Job drawing, mm, ordinate dimensions from the low corner. One solid piece. Give positions to 0.01 mm unless a question says otherwise; leave off trailing zeros. Order: outer loops, then holes, each group sorted by start corner. A loop starts at its lowest first (then second) coordinate and runs counter-clockwise, first axis right, second up. Notation, with made-up numbers: M 9,40.25 L 65,40.25 A12 ccw 65,45.25 Z; hole C -1.75,11.5 d1. An arc over 180 degrees is marked long. Put each result on its own line as item: value. Start each with the question number.
1) Drill centre lines: line 1 (Y direction, x = 46.5, z = 0.85); line 2 (X direction, y = 76, z = 0.4); line 3 (Y direction, x = 80, z = 0.75). Where is each one in solid material? Low to high. Write a range as [from, to].
2) Cut at C-C (y = 5). Write the cut outline in (x, z), and give its area (3 significant figures).
3) Cut at A-A (y = 61). Write the cut outline in (x, z).
4) Cut at B-B (x = 20). Write the cut outline in (y, z), and give its area (3 significant figures).
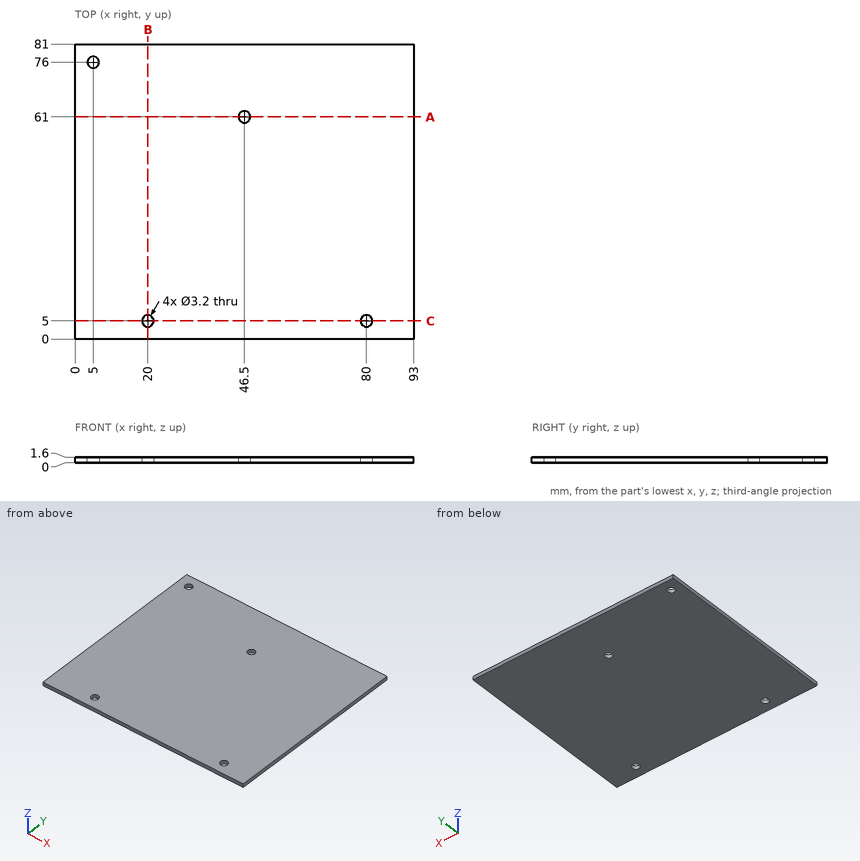
Solution:
1. line 1: [0, 59.4], [62.6, 81]
1. line 2: [0, 3.4], [6.6, 93]
1. line 3: [0, 3.4], [6.6, 81]
2. outline: M 0,0 L 18.4,0 L 18.4,1.6 L 0,1.6 Z; M 21.6,0 L 78.4,0 L 78.4,1.6 L 21.6,1.6 Z; M 81.6,0 L 93,0 L 93,1.6 L 81.6,1.6 Z
2. area: 139 mm²
3. outline: M 0,0 L 44.9,0 L 44.9,1.6 L 0,1.6 Z; M 48.1,0 L 93,0 L 93,1.6 L 48.1,1.6 Z
4. outline: M 0,0 L 3.4,0 L 3.4,1.6 L 0,1.6 Z; M 6.6,0 L 81,0 L 81,1.6 L 6.6,1.6 Z
4. area: 124 mm²
